Source: CAD feature listing. Evaluate the final solid. Frame: model axes, mm. A direction names the side the tool comes from. Coordinates: 2 decimals unless noted, no trailing zeros. Write each loop counter-clockwise with the first axis right and the second up, starting at its lowest first coordinate (ties: lowest second). Pieces come first, ordered by that corner, then holes. Notation, with made-up numbers: (-29.75, -36.5) - (6.25, -36.5) arc R27 ccw to (6.25, -10.5) - close; hole circle Ø5 at (18, -19). An arc over 180 degrees is marked (long way). One line per question, with ' | ' between items.
from build123d import *

# Parameters (mm, degrees)
F1_DEPTH       = 14
F4_D           = 6.6
F4_DEPTH       = 30
F4_CBORE_D     = 11.25
F4_CBORE_DEPTH = 20
F4_TIP         = 1.9828400428
F5_T2_ANGLE    = 203.6133668192
F5_T4_ANGLE    = 203.6133668192
F6_SIZE        = 0.5


# Not quite as in the source:
# - a fillet or chamfer that OpenCascade refuses, or shapes differently, is made with other operations: its cross-section is extruded or revolved along the edge and cut away or added


with BuildPart() as f1:
    # F0 (on Front) → F1 (new body)
    with BuildSketch(Plane.XZ):
        with BuildLine():
            Line((12.7401923062, 0), (25, 0))
            ThreePointArc((25, 0), (0, 25), (-25, 0))
            Line((-25, 0), (-12.7401923062, 0))
            ThreePointArc((-12.7401923062, 0), (0, 12.25), (12.7401923062, 0))
        make_face()
    extrude(amount=F1_DEPTH)

    # F4
    with Locations(Plane.XY.offset(25)):
        with Locations((-18.7, -7), (18.7, -7)):
            CounterBoreHole(F4_D / 2, F4_CBORE_D / 2, F4_CBORE_DEPTH, depth=F4_DEPTH)
            with Locations((0, 0, -(F4_DEPTH + F4_TIP / 2))):  # 118° drill point
                Cone(0, F4_D / 2, F4_TIP, mode=Mode.SUBTRACT)

    # F5: chamfer of 2 on 2 edges, made by hand

    # F5_s1 → F5_t2 (revolve, cut)
    with BuildSketch(Plane(origin=(0, 0, 0), x_dir=(0, 1, 0), z_dir=(-0.2046102329, 0, -0.9788435281))):
        Polygon((-12, 25), (-14, 23), (-14, 25), align=None)
    revolve(axis=Axis((0, -14, 0), (0, -1, 0)), revolution_arc=F5_T2_ANGLE, mode=Mode.SUBTRACT)

    # F5_s3 → F5_t4 (revolve, cut)
    with BuildSketch(Plane(origin=(0, 0, 0), x_dir=(0, 1, 0), z_dir=(-0.2046102329, 0, -0.9788435281))):
        Polygon((-2, 25), (0, 23), (0, 25), align=None)
    revolve(axis=Axis((0, 0, 0), (0, -1, 0)), revolution_arc=F5_T4_ANGLE, mode=Mode.SUBTRACT)

    # F6
    f6_edges = [f1.edges().sort_by_distance(p)[0] for p in [
        (0, -14, 12.25),
        (0, 0, 12.25),
    ]]
    chamfer(f6_edges, length=F6_SIZE)


solid = f1.part
Item 1: Pin query (flat end, axial travel): pin 1 Ø1 at (y, z) = (-9.5, 15.5) entering from -X; pin 2 Ø5.5 at (x, y) = (-19.5, -5) entering from +Z; pin 3 Ø1 at (y, z) = (-12, 7.5) entering from +X. Return the tip coordinate at first contact, or that it passes through.
Check sheet entries:
pin 1: x = -13.94 | pin 2: z = 5 | pin 3: x = 24
Item 2: Cut plane B-B on y = -5.75. Return loops of the section in (x, z), and give its area (3 significant figures).
Check sheet entries:
outline: (-25, 0) - (-21.75, 0) - (-21.75, 5) - (-24.18, 5) - (-24.18, 6.33) arc R25 ccw to start; (-15.65, 0) - (-12.74, 0) arc R12.75 cw to (12.74, 0) - (15.65, 0) - (15.65, 5) - (13.22, 5) - (13.22, 21.22) arc R25 ccw to (-13.22, 21.22) - (-13.22, 5) - (-15.65, 5) - close; (21.75, 0) - (25, 0) arc R25 ccw to (24.18, 6.33) - (24.18, 5) - (21.75, 5) - close | area: 441 mm²
Item 3: Cut plane C-C on y = -11.5. Return loops of the section in (x, z) (3 decimals), and give its area (3 significant figures).
Check sheet entries:
outline: (-25, 0) - (-12.74, 0) arc R12.75 cw to (12.74, 0) - (25, 0) arc R25 ccw to (22.075, 11.734) - (22.075, 5) - (15.325, 5) - (15.325, 19.752) arc R25 ccw to (-15.325, 19.752) - (-15.325, 5) - (-22.075, 5) - (-22.075, 11.734) arc R25 ccw to start | area: 586 mm²
Item 4: Mould query, pull axis X, two halves, no side actions, for faces 1 (the face through (0.513, -13.681, 23.314)), 2 (the face through (0, 0, 14)), 3 (the face through (-0.273, -6.909, 12.247)). Classes: pulls with the +X half, pulls with the -X half, needs draft (parallel to the pull), parting line crosses it, or undercut.
Check sheet entries:
face 1: parting line crosses it | face 2: needs draft | face 3: undercut
Item 5: Ray query, line 1 along Y through (x, z) = (-18.7, 12.25) (3 decimals); line 2 along Y through (x, z) = (-18.7, 3.8); line 3 along X through (y, z) = (-3.75, 8). Return the intervals inside material, ascending. Write a range as [from, to].
Check sheet entries:
line 1: [-14, -12.625], [-1.375, 0] | line 2: [-14, -10.3], [-3.7, 0] | line 3: [-23.69, -23.29], [-14.11, -9.5], [9.5, 14.11], [23.29, 23.69]
Item 6: Cut plane D-D on z = 3.5. State how many separate pieces and enclosed holes the cut face has, and give its area (3 significant figures).
Check sheet entries:
separate pieces: 2 | enclosed holes: 2 | area: 277 mm²
Item 7: Cut plane A-A on x = 0. Return loops of the section in (y, z).
Check sheet entries:
outline: (-14, 12.75) - (-13.5, 12.25) - (-0.5, 12.25) - (0, 12.75) - (0, 23) - (-2, 25) - (-12, 25) - (-14, 23) - close
Item 8: Access query for faces 4 (the face through (0, -14, 14)), 5 (the face through (-15, -7, 5)). Directions: +Z, -Z, +X, -X, +Y, -Y. A direction counts if a zero-diameter tool reaches every point of the face in a straight line with its end or side. Return the directions, or none.
Check sheet entries:
face 4: +Z, -Z, +X, -X, -Y | face 5: +Z
